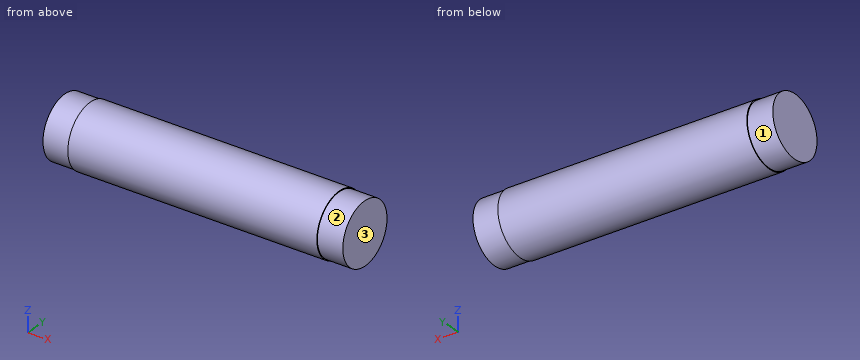
```python
from build123d import *

# Parameters (mm, degrees)
SKETCH1_R           = 6.15
BOSS_EXTRUDE1_DEPTH = 59
CUT_EXTRUDE1_START  = -5
SKETCH2_R           = 6.15
SKETCH2_R_2         = 6
CUT_EXTRUDE1_DEPTH  = 5


with BuildPart() as part:
    # Sketch1 → Boss-Extrude1 (new body)
    with BuildSketch(Plane(origin=(0, 0, 0), x_dir=(0, 0, -1), z_dir=(1, 0, 0))):
        Circle(SKETCH1_R)
    extrude(amount=BOSS_EXTRUDE1_DEPTH)

    # Sketch2 → Cut-Extrude1 (cut)
    with BuildSketch(Plane(origin=(59, 0, 0), x_dir=(0, 0, -1), z_dir=(1, 0, 0)).offset(CUT_EXTRUDE1_START)):
        Circle(SKETCH2_R)
        Circle(SKETCH2_R_2, mode=Mode.SUBTRACT)
    cut_extrude1 = extrude(amount=CUT_EXTRUDE1_DEPTH, mode=Mode.SUBTRACT)

    # Mirror1: Cut-Extrude1 across plane
    add(cut_extrude1.mirror(Plane(origin=(29.5, 0, 0), x_dir=(0, 0, 1), z_dir=(1, 0, 0))), mode=Mode.SUBTRACT)


solid = part.part
```
Input: part model. Units: mm. Frame: model coordinates. Face numbers are marked on the shaded views. A direction names the side the tool comes from. Round coordinates to 2 decimals unless told otherwise and drop trailing zeros. Loops run counter-clockwise (first coordinate to the right, second up) from the corner with the lowest first, then second, coordinate; pieces in that order, holes last. Notation, with made-up numbers: (68.5, 80.25) -> (101.5, 80.25) arc R31 cw to (101.5, 114.25) -> close; hole circle Ø7 at (64.5, 75.25). An arc over 180 degrees is marked (long way). Use one line per item in the form item = value. Start each with the question number.
Item 1: Section query D-D on x = 24. Return the cut outline in (y, z), then the cut area to 3 significant figures.
Item 2: Section query A-A on x = 4. Return the cut outline in (y, z), then the cut area to 3 significant figures.
Item 3: Contact query for a flat-ended pin moving along its axis: pin 1 Ø3 at (x, y) = (18, 4.5) entering from -Z. Output: stop coordinate, or through.
Item 4: Set-up query: the marked faces 1, 2 and 3. Return all of +Z, -Z, +X, -X, +Y, -Y with unobstructed straight access to the full face (end or side cutting, diameter ignored); none if empty.
Item 5: Section query B-B on y = -2.75. Return the cut outline in (x, z).
Item 6: Material intervals for L1, parallel to X at y = 5, z = -3.5; L2, parallel to Z at x = 27, y = -0.5; L3, parallel to Z at x = 12, y = -4, sorted ascending. Write a range as from..to.
Ans:
q1.outline = circle Ø12.3 at (0, 0)
q1.area = 119 mm^2
q2.outline = circle Ø12 at (0, 0)
q2.area = 113 mm^2
q3.pin_1 = -5.37
q4.face_1 = -X
q4.face_2 = +X
q4.face_3 = +Z, -Z, +X, +Y, -Y
q5.outline = (0, -5.33) -> (5, -5.33) -> (5, -5.5) -> (54, -5.5) -> (54, -5.33) -> (59, -5.33) -> (59, 5.33) -> (54, 5.33) -> (54, 5.5) -> (5, 5.5) -> (5, 5.33) -> (0, 5.33) -> close
q6.L1 = 5..54
q6.L2 = -6.13..6.13
q6.L3 = -4.67..4.67
